Autodesk Inventor part; units mm, degrees
ref_plane "Work Plane1" through (-1.25, 11, 0) normal (0, 0, 1) x (1, 0, 0)
ref_plane "YZ Plane" through (0, 0, 0) normal (1, 0, 0) x (0, 1, 0)
ref_plane "XZ Plane" through (0, 0, 0) normal (0, 1, 0) x (-1, 0, 0)
sketch "Sketch1" plane through (0, 0, 0) normal (0, 1, 0) x (-1, 0, 0)
  circle A0 centre (0, 0) radius 8.5
  line L0 (0, 0) -> (-2.5, 0)
  line L1 (-2.5, 0) -> (4.5, 0)
  line L2 (4.5, 0) -> (4.5, -2.5)
  line L3 (4.5, -2.5) -> (4.5, 4.5)
  line L4 (-4.5, 0) -> (-4.5, -2.5)
  line L5 (-4.5, 4.5) -> (-4.5, 0)
  line L6 (4.5, -4.5) -> (-4.5, -4.5)
  line L7 (-2.5, -2.5) -> (2.5, -2.5)
  line L8 (-2.5, -2.5) -> (-2.5, 4.5)
  line L9 (-2.5, 4.5) -> (-4.5, 4.5)
  line L10 (2.5, -2.5) -> (2.5, 4.5)
  line L11 (2.5, 4.5) -> (4.5, 4.5)
  line L12 (-4.5, -2.5) -> (-4.5, -4.5)
  line L13 (4.5, -4.5) -> (4.5, -2.5)
  point P0 (6.5, 0)
extrude "Extrusion1" add sketch "Sketch1" along normal blind 10 contours L8 L7 L10 L1 L2 L13 L6 L12 L4 L5 L9 | L10 L11 L3 L1
sketch "Sketch2" plane through (0, 10, 0) normal (0, 1, 0) x (1, 0, 0)
  circle A0 centre (0, 0) radius 8.5
  circle A1 centre (0, 0) radius 1.25
  dimension "d11" = 17
  dimension "d12" = 2.5
extrude "Extrusion2" add sketch "Sketch2" along normal blind 1
fillet "Fillet3" radius 1 1 edges at (-8.5, 10, 0)
fillet "Fillet4" radius 1 1 edges at (-1.25, 10, 0)
fillet "Fillet5" radius 6 2 edges at (3.5, 0, 4.5) (-3.5, 0, 4.5)
fillet "Fillet6" radius 10 1 edges at (0, 0, -4.5)
sketch "Sketch3" plane through (-4.5, 10, -4.5) normal (-1, 0, 0) x (0, 0, 1)
  arc A0 (3, -10) -> (9, -4) centre (3, -4) ccw
  line L0 (3, -10) -> (3, -5)
  point P0 (4.5, -10)
  dimension "d24" = 5
hole "Hole1" at (-4.5, 5, -1.5) direction (1, 0, 0) diameter 4 depth 10
sketch "Sketch4" plane through (2.5, 10, -2.5) normal (-1, 0, 0) x (0, 0, 1)
  line L0 (7, -4) -> (7, 0)
  circle A0 centre (3.75, -7) radius 1.25
  point P0 (2.5, -10)
extrude "Extrusion3" add sketch "Sketch4" along normal blind 2.5
chamfer "Chamfer1" distance 0.25 distance2 1.25 1 edges at (0, 3, 0) measured on face at (0, 2.3808, 1.5915)
sketch "Sketch5" plane through (-2.5, 10, 4.5) normal (1, 0, 0) x (0, 0, -1)
  circle A0 centre (3.25, -7) radius 1.25
  circle A1 centre (3.25, -7) radius 1.25
  point P0 (4.5, -10)
extrude "Extrusion4" add sketch "Sketch5" along normal blind 2.5
chamfer "Chamfer2" distance 0.25 distance2 1.25 1 edges at (0, 3, 2.5) measured on face at (0, 2.8205, 0.1051)
ref_plane "Work Plane1" through (-1.25, 11, 0) normal (0, 0, 1) x (1, 0, 0)
sketch "Sketch7" plane through (-1.25, 11, 0) normal (0, 0, 1) x (1, 0, 0)
  line L0 (0, 0) -> (2.5, 0)
  line L1 (1.25, 0) -> (1.25, 25)
  line L2 (1.25, 0) -> (1.25, 24)
  line L3 (1.25, 24) -> (6.0871, 24) construction
  line L4 (6.0871, 24) -> (8.9052, 17.9211) construction
  line L5 (9.75, 0) -> (-7.25, 0)
  line L6 (8.9052, 17.9211) -> (9.75, 0) construction
  spline S0 degree 3 poles (1.25, 24) (6.0871, 24) (8.9052, 17.9211) (9.75, 0) knots 1 1 1 1 2 2 2 2
  line L7 (9.75, 0) -> (1.25, 0)
  point P0 (1.25, -11)
  dimension "d48" = 25
  dimension "d49" = 24
revolve "Revolution1" add sketch "Sketch7" angle 360 about axis through (0, 11, 0) along (0, 1, 0)
sketch "Sketch8" plane through (0, 11, 0) normal (0, -1, 0) x (1, 0, 0)
  circle A0 centre (0, 0) radius 1.25
hole "Hole2" at (0, 11, 0) direction (0, 1, 0) diameter 1 depth 40
fillet "Fillet7" radius 1 1 edges at (0, 11, 0.5)
properties part number "Index_3" material "ABS Plastic"
Geometry check sheet. Reference: the model listing, model coordinates, mm. A direction names the side the tool comes from. Give positions to 0.01 mm unless a question says otherwise; leave off trailing zeros. Write each loop counter-clockwise with the first axis right and the second up, starting at its lowest first coordinate (ties: lowest second). Pieces come first, ordered by that corner, then holes.
1) Cross-section at A-A (y = 5). Record the boundary of the cut face in (x, z).
Values follow:
outline: (-4.5, -4.45) - (4.5, -4.45) - (4.5, -3.5) - (-4.5, -3.5) - close; (-4.5, 0.5) - (-2.5, 0.5) - (-2.5, 4.42) - (-4.5, 4.42) - close; (2.5, 0.5) - (4.5, 0.5) - (4.5, 4.42) - (2.5, 4.42) - close
2) Release check for a two-part mould opening along Y. For faces 1 (the face through (1.884, 2.155, 0.329)), 2 (the face through (0, 8, -2.5)), 3 (the face through (-3, 0, -2)) record: released by +Y, released by -Y, zero draft, split by the parting line, or undercut.
Values follow:
face 1: undercut
face 2: zero draft
face 3: released by -Y
3) Set-up check for faces 4 (the face through (-3, 8, 4.5)), 5 (the face through (0.488, 23.634, 0.108)), 6 (the face through (4.5, 6, 1)), 7 (the face through (0, 2, -2.5)), 8 (the face through (-2, 3, 0)): record each of +Z, -Z, +X, -X, +Y, -Y from which the full face is reachable in a straight line by a thin tool's end or side.
Values follow:
face 4: +Z, +X, -X, -Y
face 5: +Y
face 6: +Z, -Z, +X, -Y
face 7: -Y
face 8: none
4) Thickness scan on line 1 (X direction, y = 2.5, z = 3.25); line 2 (Z direction, x = 0, y = 24.25); line 3 (Z direction, x = -1, y = 4). Record the ranges inside material, lowest first.
Values follow:
line 1: x = -4.5 to -2.5, 2.5 to 4.5
line 2: z = -7.18 to -0.5, 0.5 to 7.18
line 3: z = -4.3 to -3.23, 0.59 to 1.91
5) Go/stop test with flat-tipped pins: pin 1 Ø1.6 at (x, y) = (1, 1.5) entering from +Z; pin 2 Ø4.5 at (y, z) = (6.5, 1.5) entering from -X; pin 3 Ø5 at (x, z) = (-1, 1.5) entering from -Y; pin 4 Ø3 at (y, z) = (5, -1.5) entering from -X. Record where each tip stops, or that it passes through.
Values follow:
pin 1: stops at z = 2.26
pin 2: stops at x = -4.5
pin 3: stops at y = 0.08
pin 4: passes through
